```python
from build123d import *

# Parameters (mm, degrees)
SKETCH1_R           = 2.6
BOSS_EXTRUDE1_DEPTH = 20
SKETCH2_R           = 2.6
CUT_EXTRUDE1_DEPTH  = 20
CUT_EXTRUDE2_DEPTH  = 3
CUT_EXTRUDE3_DEPTH  = 8
FILLET1_R           = 1


with BuildPart() as part:
    # Sketch1 → Boss-Extrude1 (new body)
    with BuildSketch(Plane.XY):
        with BuildLine():
            Line((-30, 0), (30, 0))
            Line((30, 0), (30, -15))
            ThreePointArc((30, -15), (28.535533906, -18.535533906), (25, -20))
            Line((25, -20), (-25, -20))
            ThreePointArc((-25, -20), (-28.535533906, -18.535533906), (-30, -15))
            Line((-30, -15), (-30, 0))
        make_face()
        with Locations((0, -10)):
            Circle(SKETCH1_R, mode=Mode.SUBTRACT)
    extrude(amount=BOSS_EXTRUDE1_DEPTH)

    # Sketch2 → Cut-Extrude1 (cut)
    with BuildSketch(Plane(origin=(0, 0, 0), x_dir=(1, 0, 0), z_dir=(0, 1, 0))):
        with Locations(Location((-20, -10, 0), (0, 0, 180))):
            Circle(SKETCH2_R)
        with Locations(Location((20, -10, 0), (0, 0, 180))):
            Circle(SKETCH2_R)
    extrude(amount=-CUT_EXTRUDE1_DEPTH, mode=Mode.SUBTRACT)

    # Sketch3 → Cut-Extrude2 (cut)
    with BuildSketch(Plane(origin=(0, 0, 0), x_dir=(-1, 0, 0), z_dir=(0, 0, -1))):
        Polygon((6.062177826, -10), (3.031088913, -4.75), (-3.031088913, -4.75), (-6.062177826, -10), (-3.031088913, -15.25), (3.031088913, -15.25), align=None)
    extrude(amount=-CUT_EXTRUDE2_DEPTH, mode=Mode.SUBTRACT)

    # Sketch4 → Cut-Extrude3 (cut)
    with BuildSketch(Plane.XY.offset(20)):
        Polygon((-4, -7.690598923), (-4, -12.309401077), (0, -14.618802154), (4, -12.309401077), (4, -7.690598923), (0, -5.381197846), align=None)
    extrude(amount=-CUT_EXTRUDE3_DEPTH, mode=Mode.SUBTRACT)

    # Fillet1
    fillet1_edges = [part.edges().sort_by_distance(p)[0] for p in [
        (0, -20, 20),
        (28.535533906, -18.535533906, 20),
        (30, -7.5, 20),
        (-30, -7.5, 20),
        (30, -7.5, 0),
        (28.535533906, -18.535533906, 0),
        (-28.535533906, -18.535533906, 20),
        (0, -20, 0),
        (-28.535533906, -18.535533906, 0),
        (-30, -7.5, 0),
    ]]
    fillet(fillet1_edges, radius=FILLET1_R)


solid = part.part
```
Geometry check sheet. Reference: the model listing, model coordinates, mm. A direction names the side the tool comes from. Round coordinates to 2 decimals unless told otherwise and drop trailing zeros. Write each loop counter-clockwise with the first axis right and the second up, starting at its lowest first coordinate (ties: lowest second). Pieces come first, ordered by that corner, then holes. Notation, with made-up numbers: (-13, 20.25) -> (29, 20.25) arc R3 cw to (29, 24.25) -> close; hole circle Ø1 at (29, 13). An arc over 180 degrees is marked (long way). Put each result on its own line as item: value.
1) Cross-section at B-B, the plane z = 14.75. Enter the section's corners in (x, y), plus the area to 3 significant figures.
Recorded:
outline: (-30, -15) arc R5 ccw to (-25, -20) -> (25, -20) arc R5 ccw to (30, -15) -> (30, 0) -> (-30, 0) -> close; hole (-4, -12.31) -> (0, -14.62) -> (4, -12.31) -> (4, -7.69) -> (0, -5.38) -> (-4, -7.69) -> close
area: 1,130 mm2
2) Cross-section at A-A, the plane z = 10. Enter the section's corners in (x, y), plus the area to 3 significant figures.
Recorded:
outline: (-30, -15) arc R5 ccw to (-25, -20) -> (-22.6, -20) -> (-22.6, 0) -> (-30, 0) -> close; (-17.4, -20) -> (17.4, -20) -> (17.4, 0) -> (-17.4, 0) -> close; (22.6, -20) -> (25, -20) arc R5 ccw to (30, -15) -> (30, 0) -> (22.6, 0) -> close; hole circle Ø5.2 at (0, -10)
area: 960 mm2
3) Thickness scan on probe 1 along Z at (x, y) = (20, -12.5); probe 2 along X at (y, z) = (-6.5, 8.25); probe 3 along Y at (x, z) = (0, 6.5). Record the ranges inside material, lowest first. Write a range as from..to.
Recorded:
probe 1: z = 0..7.4, 12.6..20
probe 2: x = -30..-21.92, -18.08..18.08, 21.92..30
probe 3: y = -20..-12.6, -7.4..0
4) Cross-section at D-D, the plane z = 6.5. Enter the section's corners in (x, y).
Recorded:
outline: (-30, -15) arc R5 ccw to (-25, -20) -> (25, -20) arc R5 ccw to (30, -15) -> (30, 0) -> (-30, 0) -> close; hole circle Ø5.2 at (0, -10)
5) Depth check by flat-ended pin: P1, Ø3, axis at x = 20, z = 10, coming from the -Y side; P2, Ø3, axis at x = 1.5, y = -10, coming from the -Z side. Enter the tip coordinate at first touch or a pass-through.
Recorded:
P1: passes through
P2: stops at z = 3
6) Cross-section at C-C, the plane x = -1. Enter the section's corners in (y, z).
Recorded:
outline: (-20, 1) arc R1 ccw to (-19, 0) -> (-15.25, 0) -> (-15.25, 3) -> (-12.4, 3) -> (-12.4, 12) -> (-14.04, 12) -> (-14.04, 20) -> (-19, 20) arc R1 ccw to (-20, 19) -> close; (-7.6, 3) -> (-4.75, 3) -> (-4.75, 0) -> (0, 0) -> (0, 20) -> (-5.96, 20) -> (-5.96, 12) -> (-7.6, 12) -> close
7) Release check for a two-part mould opening along Y. For faces 4 (the face through (4.568, -12.588, 1.479)), 5 (the face through (0, 0, 10)), 6 (the face through (-0.56, -12.54, 7.44)), 7 (the face through (29, -18, 10)) record: pulls with the +Y half, pulls with the -Y half, needs draft (parallel to the pull), parting line crosses it, or undercut.
Recorded:
face 4: undercut
face 5: pulls with the +Y half
face 6: undercut
face 7: pulls with the -Y half
8) Access from +Z, -Z, +X, -X, +Y, -Y to the whole of each face (thin tool, end or side, straight path). Record for faces 1 (the face through (0, -5, 20)), 2 (the face through (-4, -10, 16)), 3 (the face through (0, -15.25, 1)).
Recorded:
face 1: +Z, +X, -X, +Y, -Y
face 2: +Z
face 3: -Z
